Read the model definition and answer for the solid it produces. Units are mm, in the model's axes. Face numbers are marked on the shaded views. A direction names the side the tool comes from. Coordinates: 2 decimals unless noted, no trailing zeros. Write each loop counter-clockwise with the first axis right and the second up, starting at its lowest first coordinate (ties: lowest second). Pieces come first, ordered by that corner, then holes.
(1) Which of the six approach directions +Z, -Z, +X, -X, +Y, -Y give full straight-line access (tool end or side, diameter ignored) to the marked faces 1 and 2?
(2) Given pin 1 (0.8 mm diameter, centred on x = 103.5, y = 0.5, fed in from +Z); pin 2 (1.7 mm diameter, centred on x = 7, z = -85, fed in from +Y); pin 3 (4 mm diameter, centred on x = 86, z = -63.5, fed in from -Y); pin 4 (1 mm diameter, centred on y = -2, z = -79, fed in from -X), each flat-ended and moving along its own axis, determine where each tip first touches the part or whether it passes through.
(3) Section A-A on y = -3.5 is taken. Write down the section's boundary in (x, z).
(4) Find the intervals of material crossed by probe 1 along Z at (x, y) = (6, -1.95); probe 2 along X at (y, z) = (0.2, -15); probe 3 along Y at (x, z) = (105, -44), in increasing order.
(5) Section D-D on x = 134 is taken. Write down the section's boundary in (y, z).
(6) Section C-C on x = 104.5 is taken. Write down the section's boundary in (y, z), then the cut area to 3 significant figures.
(7) Section B-B on z = -6.5 is taken. Write down the section's boundary in (x, y), then the cut area to 3 significant figures.
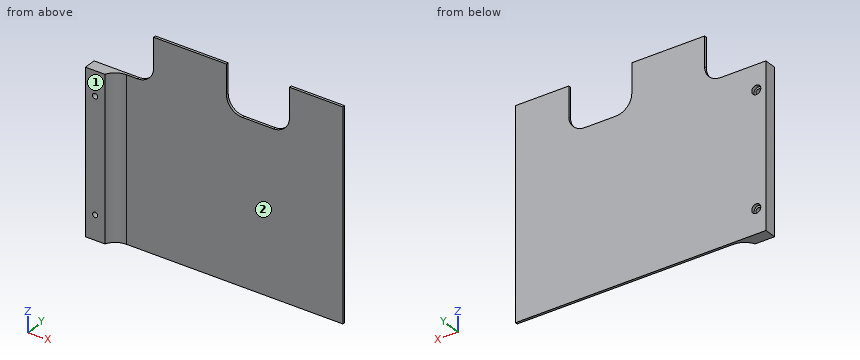
from build123d import *

# Parameters (mm, degrees)
CROQUIS1_W              = 155
CROQUIS1_H              = 100
SALIENTE_EXTRUIR1_DEPTH = 1.5
CROQUIS2_R              = 1.6
CORTAR_EXTRUIR1_DEPTH   = 1.5
CROQUIS3_W              = 12
CROQUIS3_H              = 100
CROQUIS3_R              = 1.6
SALIENTE_EXTRUIR2_DEPTH = 6
CROQUIS4_W              = 45
CROQUIS4_H              = 28
CROQUIS4_W_2            = 33
SALIENTE_EXTRUIR3_DEPTH = 1.5
REDONDEO1_R             = 10
REDONDEO2_R             = 10
CROQUIS5_R              = 2.8
CORTAR_EXTRUIR2_DEPTH   = 2


with BuildPart() as part:
    # Croquis1 → Saliente-Extruir1 (new body)
    with BuildSketch(Plane(origin=(0, 0, 0), x_dir=(1, 0, 0), z_dir=(0, 1, 0))):
        with Locations((77.5, 50)):
            Rectangle(CROQUIS1_W, CROQUIS1_H)
    extrude(amount=SALIENTE_EXTRUIR1_DEPTH)

    # Croquis2 → Cortar-Extruir1 (cut)
    with BuildSketch(Plane(origin=(0, 1.5, 0), x_dir=(1, 0, 0), z_dir=(0, 1, 0))):
        with Locations(Location((6, 85, 0), (0, 0, 270))):
            Circle(CROQUIS2_R)
        with Locations(Location((6, 15, 0), (0, 0, 270))):
            Circle(CROQUIS2_R)
    extrude(amount=-CORTAR_EXTRUIR1_DEPTH, mode=Mode.SUBTRACT)

    # Croquis3 → Saliente-Extruir2 (add)
    with BuildSketch(Plane.XZ):
        with Locations((6, -50)):
            Rectangle(CROQUIS3_W, CROQUIS3_H)
        with Locations(Location((6, -15, 0), (0, 0, 90))):
            Circle(CROQUIS3_R, mode=Mode.SUBTRACT)
        with Locations(Location((6, -85, 0), (0, 0, 90))):
            Circle(CROQUIS3_R, mode=Mode.SUBTRACT)
    extrude(amount=SALIENTE_EXTRUIR2_DEPTH)

    # Croquis4 → Saliente-Extruir3 (add)
    with BuildSketch(Plane(origin=(0, 1.5, 0), x_dir=(1, 0, 0), z_dir=(0, 1, 0))):
        with Locations((60.5, -14)):
            Rectangle(CROQUIS4_W, CROQUIS4_H)
        with Locations((138.5, -14)):
            Rectangle(CROQUIS4_W_2, CROQUIS4_H)
    extrude(amount=-SALIENTE_EXTRUIR3_DEPTH)

    # Redondeo1
    redondeo1_edges = [part.edges().sort_by_distance(p)[0] for p in [
        (83, 0.75, 0),
        (38, 0.75, 0),
        (122, 0.75, 0),
    ]]
    fillet(redondeo1_edges, radius=REDONDEO1_R)

    # Redondeo2
    # the kernel refuses this fillet: 10 mm, written as the material it adds along each edge
    with BuildSketch(Plane(origin=(12, 0, -100), x_dir=(0, -1, 0), z_dir=(0, 0, 1))) as redondeo2_piece_1:
        with BuildLine():
            CenterArc((10, 9.16515139), REDONDEO2_R, 180, 66.421821522)
            Line((0, 9.16515139), (-0.2, 9.16515139))
            Line((-0.2, 9.16515139), (-0.2, 0))
            Line((-0.2, 0), (0, -0.2))
            ThreePointArc((0, -0.2), (3, -0.2), (5.92, -0.183303028))
            Line((5.92, -0.183303028), (6, 0))
        make_face()
    extrude(amount=100)

    # Croquis5 → Cortar-Extruir2 (cut)
    with BuildSketch(Plane(origin=(0, 1.5, 0), x_dir=(1, 0, 0), z_dir=(0, 1, 0))):
        with Locations(Location((6, 85, 0), (0, 0, 270))):
            Circle(CROQUIS5_R)
        with Locations(Location((6, 15, 0), (0, 0, 270))):
            Circle(CROQUIS5_R)
    extrude(amount=-CORTAR_EXTRUIR2_DEPTH, mode=Mode.SUBTRACT)


solid = part.part
Response:
1. face 1: +Z, -Z, +X, -X, -Y
1. face 2: +Z, -Z, +X, -Y
2. pin 1: stops at z = 0
2. pin 2: stops at y = -0.5
2. pin 3: stops at y = 0
2. pin 4: stops at x = 0
3. outline: (0, -100) - (13.57, -100) - (13.57, 0) - (0, 0) - close; hole circle Ø3.2 at (6, -85); hole circle Ø3.2 at (6, -15)
4. probe 1: z = -100 to -86.6, -83.4 to -16.6, -13.4 to 0
4. probe 2: x = 0 to 3.2, 8.8 to 155
4. probe 3: y = 0 to 1.5
5. outline: (0, -100) - (1.5, -100) - (1.5, 28) - (0, 28) - close
6. outline: (0, -100) - (1.5, -100) - (1.5, 0) - (0, 0) - close
6. area: 150 mm2
7. outline: (0, -6) - (12, -6) arc R10 cw to (21.17, 0) - (155, 0) - (155, 1.5) - (0, 1.5) - close
7. area: 320 mm2
